from build123d import *

# Parameters (mm, degrees)
BASE_FLANGE1_DEPTH = 10
SKETCH7_R          = 1.5875
CUT_EXTRUDE1_DEPTH = 31.822070015
SKETCH8_R          = 1.984375
CUT_EXTRUDE2_DEPTH = 31.822070015
FILLET1_R          = 3


# Sheet-metal steps are written as plain solids
with BuildPart() as part:
    # Sketch2 → Base-Flange1 (new, symmetric)
    with BuildSketch(Plane.XY):
        with BuildLine():
            Line((0, 25), (0, 0.7366))
            ThreePointArc((0, 0.7366), (0.215745145, 0.215745145), (0.7366, 0))
            Line((0.7366, 0), (15, 0))
            Line((15, 0), (15, -0.7366))
            Line((15, -0.7366), (0.7366, -0.7366))
            ThreePointArc((0.7366, -0.7366), (-0.30510971, -0.30510971), (-0.7366, 0.7366))
            Line((-0.7366, 0.7366), (-0.7366, 25))
            Line((-0.7366, 25), (0, 25))
        make_face()
    extrude(amount=BASE_FLANGE1_DEPTH, both=True)

    # Sketch7 → Cut-Extrude1 (cut, through all)
    with BuildSketch(Plane(origin=(0, 0, 0), x_dir=(0, 0, -1), z_dir=(1, 0, 0))):
        with Locations(Location((0.42, 12.4934, 0), (0, 0, 90))):
            Circle(SKETCH7_R)
    extrude(amount=-CUT_EXTRUDE1_DEPTH, mode=Mode.SUBTRACT)

    # Sketch8 → Cut-Extrude2 (cut, through all)
    with BuildSketch(Plane(origin=(0, 0, 0), x_dir=(1, 0, 0), z_dir=(0, 1, 0))):
        with Locations(Location((10, 0, 0), (0, 0, 270))):
            Circle(SKETCH8_R)
    extrude(amount=-CUT_EXTRUDE2_DEPTH, mode=Mode.SUBTRACT)

    # Fillet1
    fillet1_edges = [part.edges().sort_by_distance(p)[0] for p in [
        (-0.3683, 25, 10),
        (-0.3683, 25, -10),
    ]]
    fillet(fillet1_edges, radius=FILLET1_R)


solid = part.part
Build history of the part. All positions in model axes, mm. A direction names the side the tool comes from. Round coordinates to 2 decimals unless told otherwise and drop trailing zeros. Write each loop counter-clockwise with the first axis right and the second up, starting at its lowest first coordinate (ties: lowest second). Pieces come first, ordered by that corner, then holes. Notation, with made-up numbers: (83, -13) -> (92, -13) arc R21 cw to (92, 25) -> close; hole circle Ø5 at (22, -17.75). An arc over 180 degrees is marked (long way). Write item = value, one per line.
(1) Probe L1, parallel to Y at x = 2.75, z = 2.75; L2, parallel to X at y = -0.15, z = 0. List the from-to ranges inside material, lowest first.
Answer:
L1 = -0.74 to 0
L2 = -0.44 to 8.02, 11.98 to 15
(2) Tool access for faces 1 (the face through (7.8, 0, 0.1)), 2 (the face through (-0.36, 24.14, -9.1)): list every direction of +Z, -Z, +X, -X, +Y, -Y with a clear straight run to the whole face (end or side of a thin tool).
Answer:
face_1 = +Z, -Z, +X, +Y
face_2 = -Z, +X, -X, +Y
(3) Band-saw the part on D-D (z = 8.5). Give the cut face in (x, y).
Answer:
outline = (-0.74, 0.74) arc R1.47 ccw to (0.74, -0.74) -> (15, -0.74) -> (15, 0) -> (0.74, 0) arc R0.74 cw to (0, 0.74) -> (0, 24.6) -> (-0.74, 24.6) -> close
(4) Band-saw the part on A-A (x = 10). Give the cut face in (y, z), then the cut area to 3 significant figures.
Answer:
outline = (-0.74, -10) -> (0, -10) -> (0, -1.98) -> (-0.74, -1.98) -> close; (-0.74, 1.98) -> (0, 1.98) -> (0, 10) -> (-0.74, 10) -> close
area = 11.8 mm2
(5) Band-saw the part on C-C (y = 13.75). Give the cut face in (x, z).
Answer:
outline = (-0.74, -10) -> (0, -10) -> (0, -1.39) -> (-0.74, -1.39) -> close; (-0.74, 0.55) -> (0, 0.55) -> (0, 10) -> (-0.74, 10) -> close
(6) Flat gauge pins, fed straight in: pin 1 (4.5 mm diameter, centred on x = 8.5, z = -4.5, fed in from +Y); pin 2 (1 mm diameter, centred on y = 12.5, z = 4.5, fed in from +X). Where does each tip first touch, or does it go through?
Answer:
pin_1 = 0
pin_2 = 0
(7) Two-plate mould, pull along X, no slides. Class faces 3 (the face through (-0.737, 13, 2)), 4 (the face through (0, 13, 2)), 5 (the face through (-0.36, 24.14, 9.1)), 6 (the face through (8.063, -0.363, -0.43)): pulls with the +X half, pulls with the -X half, needs draft (parallel to the pull), parting line crosses it, or undercut.
Answer:
face_3 = pulls with the -X half
face_4 = pulls with the +X half
face_5 = needs draft
face_6 = undercut
(8) Band-saw the part on B-B (z = 0). Give the cut face in (x, y), then the cut area to 3 significant figures.
Answer:
outline = (-0.74, 0.74) arc R1.47 ccw to (0.74, -0.74) -> (8.02, -0.74) -> (8.02, 0) -> (0.74, 0) arc R0.74 cw to (0, 0.74) -> (0, 10.96) -> (-0.74, 10.96) -> close; (-0.74, 14.02) -> (0, 14.02) -> (0, 25) -> (-0.74, 25) -> close; (11.98, -0.74) -> (15, -0.74) -> (15, 0) -> (11.98, 0) -> close
area = 24.5 mm2
